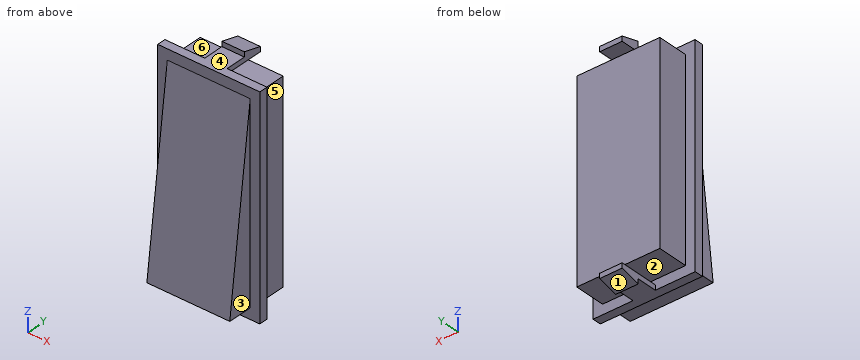
```python
from build123d import *

# Parameters (mm, degrees)
SKETCH1_W           = 24.13
SKETCH1_H           = 50.7
BOSS_EXTRUDE1_DEPTH = 2.02
SKETCH2_W           = 19.6
SKETCH2_H           = 46.08
BOSS_EXTRUDE2_DEPTH = 7.29
BOSS_EXTRUDE3_START = -2.265
BOSS_EXTRUDE3_DEPTH = 19.6
SKETCH4_W           = 5.3
SKETCH4_H           = 9.38
BOSS_EXTRUDE4_DEPTH = 1.155
BOSS_EXTRUDE5_DEPTH = 5.3


with BuildPart() as part:
    # Sketch1 → Boss-Extrude1 (new body)
    with BuildSketch(Plane(origin=(0, 0, 0), x_dir=(1, 0, 0), z_dir=(0, 1, 0))):
        Rectangle(SKETCH1_W, SKETCH1_H)
    extrude(amount=BOSS_EXTRUDE1_DEPTH)

    # Sketch2 → Boss-Extrude2 (add)
    with BuildSketch(Plane(origin=(0, 2.02, 0), x_dir=(1, 0, 0), z_dir=(0, 1, 0))):
        Rectangle(SKETCH2_W, SKETCH2_H)
    extrude(amount=BOSS_EXTRUDE2_DEPTH)

    # Sketch3 → Boss-Extrude3 (add)
    with BuildSketch(Plane(origin=(12.065, 0, 0), x_dir=(0, 0, -1), z_dir=(1, 0, 0)).offset(BOSS_EXTRUDE3_START)):
        Polygon((-22.884943392, 0), (22.781251072, -5.781035599), (22.781251072, 0), align=None)
    extrude(amount=-BOSS_EXTRUDE3_DEPTH)

    # Sketch4 → Boss-Extrude4 (add)
    with BuildSketch(Plane(origin=(0, 0, -25.35), x_dir=(-1, 0, 0), z_dir=(0, 0, -1))):
        with Locations((0, 6.71)):
            Rectangle(SKETCH4_W, SKETCH4_H)
    boss_extrude4 = extrude(amount=-BOSS_EXTRUDE4_DEPTH)

    # Sketch5 → Boss-Extrude5 (add)
    with BuildSketch(Plane(origin=(2.65, 0, 0), x_dir=(0, 0, -1), z_dir=(1, 0, 0))):
        Polygon((25.35, 11.4), (25.35, 6.9), (26.51, 6.9), align=None)
    boss_extrude5 = extrude(amount=-BOSS_EXTRUDE5_DEPTH)

    # Mirror1: Boss-Extrude4, Boss-Extrude5 across plane
    add(boss_extrude4.mirror(Plane.XY))
    add(boss_extrude5.mirror(Plane.XY))


solid = part.part
```
Check sheet for the modelled part. Datum: model origin and axes. Units: mm. Face numbers are marked on the shaded views. A direction names the side the tool comes from. Round coordinates to 2 decimals unless told otherwise and drop trailing zeros. Loops run counter-clockwise (first coordinate to the right, second up) from the corner with the lowest first, then second, coordinate; pieces in that order, holes last. Notation, with made-up numbers: M 79,43 L 131,43 A23 cw 131,56 Z; hole C 45,45.5 d11. An arc over 180 degrees is marked long. Answer as a JSON object with one key per item and string values.
1. Scan lines: line 1 (Z direction, x = 1.5, y = 3) (3 decimals); line 2 (Y direction, x = -10.25, z = 14); line 3 (X direction, y = -1.75, z = 6). Record each from-to range of solid material in increasing order.
Reply:
{"line 1": "z = -25.35 to -24.195, -23.04 to 23.04, 24.195 to 25.35", "line 2": "y = 0 to 2.02", "line 3": "x = -9.8 to 9.8"}
2. Section check C-C (z = 0.5). Record the boundary of the cut face in (x, y) (3 decimals).
Reply:
{"outline": "M -12.065,0 L -9.8,0 L -9.8,-2.834 L 9.8,-2.834 L 9.8,0 L 12.065,0 L 12.065,2.02 L 9.8,2.02 L 9.8,9.31 L -9.8,9.31 L -9.8,2.02 L -12.065,2.02 Z"}
3. Section check B-B (x = 0). Record the boundary of the cut face in (y, z) (3 decimals).
Reply:
{"outline": "M -5.781,-22.781 L 0,-22.781 L 0,-25.35 L 6.9,-25.35 L 6.9,-26.51 L 11.4,-25.35 L 11.4,-24.195 L 2.02,-24.195 L 2.02,-23.04 L 9.31,-23.04 L 9.31,23.04 L 2.02,23.04 L 2.02,24.195 L 11.4,24.195 L 11.4,25.35 L 6.9,26.51 L 6.9,25.35 L 0,25.35 L 0,22.885 Z"}
4. Section check A-A (y = 3.25). Record the boundary of the cut face in (x, z) (3 decimals).
Reply:
{"outline": "M -9.8,-23.04 L 9.8,-23.04 L 9.8,23.04 L -9.8,23.04 Z; M -2.65,-25.35 L 2.65,-25.35 L 2.65,-24.195 L -2.65,-24.195 Z; M -2.65,24.195 L 2.65,24.195 L 2.65,25.35 L -2.65,25.35 Z"}
5. Access from +Z, -Z, +X, -X, +Y, -Y to the whole of each face (thin tool, end or side, straight path). Record for the marked faces 4, 5 and 6.
Reply:
{"face 4": "+Z, +X, -X, -Y", "face 5": "+Z, -Z, +X, +Y", "face 6": "+X, -X, +Y"}
6. Gauge pin test, flat ends, axial feed: P1, Ø1.7, axis at y = -3, z = -1.5, coming from the -X side; P2, Ø6, axis at x = -0.5, y = 4.5, coming from the +Z side; P3, Ø5, axis at x = -7.5, y = 9.5, coming from the -Z side; P4, Ø1.5, axis at x = 5.5, z = -19.5, coming from the -Y side. Record the tip position at first contact, or that the pin passes through.
Reply:
{"P1": "stops at x = -9.8", "P2": "stops at z = 26.51", "P3": "stops at z = -23.04", "P4": "stops at y = -5.46"}
7. Mould release check, pull along Z, two halves, no side actions. Record for the marked faces 1, 2 and 3: pulls with the +Z half, pulls with the -Z half, needs draft (parallel to the pull), parting line crosses it, or undercut.
Reply:
{"face 1": "pulls with the -Z half", "face 2": "undercut", "face 3": "needs draft"}
8. Section check D-D (y = 0.5). Record the boundary of the cut face in (x, z) (3 decimals), plus the area to 3 significant figures.
Reply:
{"outline": "M -12.065,-25.35 L 12.065,-25.35 L 12.065,25.35 L -12.065,25.35 Z", "area": "1,220 mm²"}
